Print and shaded views of the part. All mm, measured from the part's lowest x, y and z. Round coordinates to 2 decimals unless told otherwise and drop trailing zeros. Order: outer loops, then holes, each group sorted by start corner. A loop starts at its lowest first (then second) coordinate and runs counter-clockwise, first axis right, second up. Notation, with made-up numbers: M 23,70 L 31,70 A27 cw 31,97 Z; hole C 86.25,44 d6. An arc over 180 degrees is marked long. Write each question's results on one line, items separated by ' | '. Start each with the question number.
1. Drop flat-ended pins along their axis: pin 1 Ø10 at (y, z) = (24, 66.5) entering from +X; pin 2 Ø6 at (x, z) = (23.5, 51.5) entering from +Y; pin 3 Ø12 at (x, z) = (30, 73.5) entering from +Y. Give the stop position or say it passes through.
2. Band-saw the part on A-A, the plane z = 30.5. List the corners of the cut face in (x, y).
3. Probe L1, parallel to Z at x = 8, y = 31.5; L2, parallel to Y at x = 18, z = 35; L3, parallel to Y at x = 29, z = 80. List the from-to ranges inside material, lowest first. Write a range as [from, to].
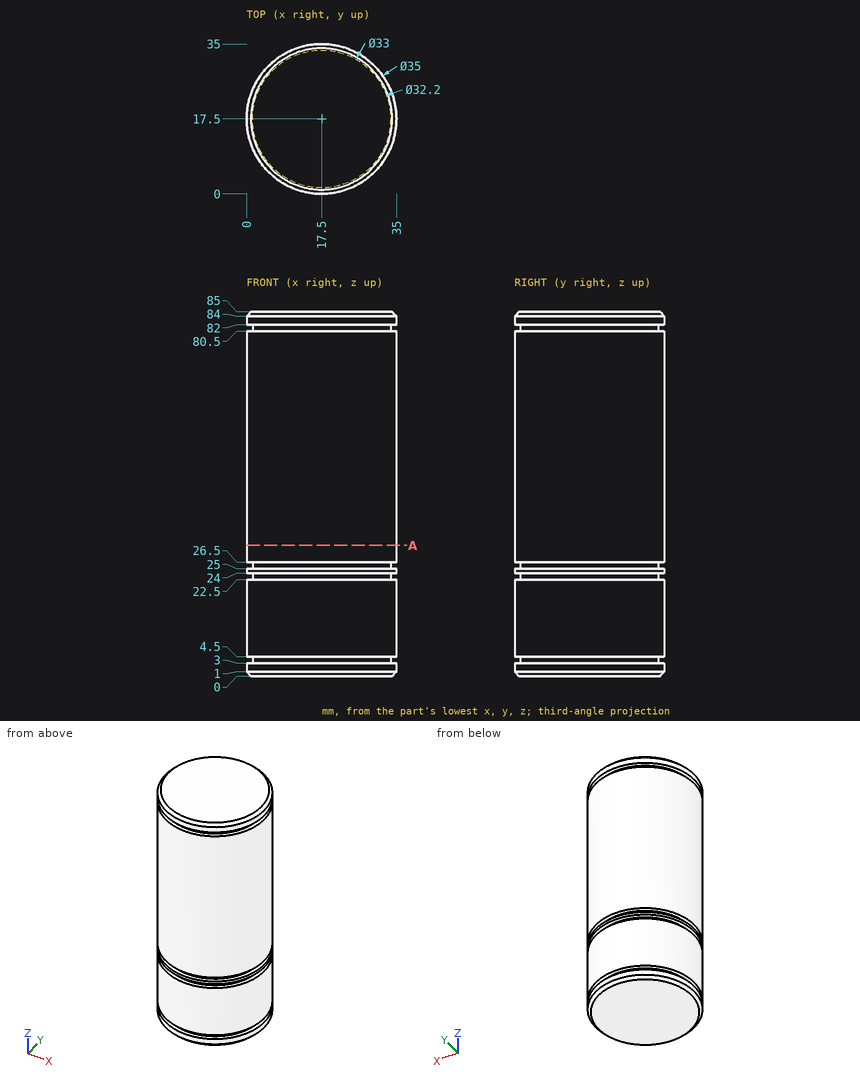
Solution:
1) pin 1: x = 34.94 | pin 2: y = 34.74 | pin 3: y = 33.75
2) outline: C 17.5,17.5 d35
3) L1: [0.42, 3], [4.5, 22.5], [24, 25], [26.5, 80.5], [82, 84.58] | L2: [0.01, 34.99] | L3: [4.31, 30.69]
